```python
from build123d import *

# Parameters (mm, degrees)
GEARFACEPROFILE_R        = 15
GEARFACEEXTRUDE_DEPTH    = 12.21
CENTERSLOT_DEPTH         = 25.476194557
GEARCONNECTORS_OUTLINE_R = 3.5
GEARCONNECTORS_DEPTH     = 3.8
SETSCREWPROFILE_R        = 2.52
SETSCREWHOLE_DEPTH       = 25.476194557


# Read off the part's stored shape, not the designer's step: GearConnectors
with BuildPart() as part:
    # GearFaceProfile → GearFaceExtrude (new body)
    with BuildSketch(Plane.XY):
        Circle(GEARFACEPROFILE_R)
    extrude(amount=GEARFACEEXTRUDE_DEPTH)

    # Sketch1 → CenterSlot (cut, through all)
    with BuildSketch(Plane.XY.offset(12.21)):
        with BuildLine():
            Line((-1.335, 6.504411964), (-1.335, 4.704411964))
            Line((-1.335, 4.704411964), (1.335, 4.704411964))
            Line((1.335, 4.704411964), (1.335, 6.504411964))
            ThreePointArc((1.335, 6.504411964), (0, -6.64), (-1.335, 6.504411964))
        make_face()
    extrude(amount=-CENTERSLOT_DEPTH, mode=Mode.SUBTRACT)

    # GearConnectors outline → GearConnectors (add)
    with BuildSketch(Plane(origin=(0, 0, 0), x_dir=(-1, 0, 0), z_dir=(0, 0, -1))):
        with BuildLine():
            ThreePointArc((5.310262334, -3.986315836), (11.691342952, -6.749999998), (6.107381948, -2.605664164))
            ThreePointArc((6.107381948, -2.605664164), (5.750408681, -3.32), (5.310262334, -3.986315836))
        make_face()
        with BuildLine():
            ThreePointArc((-6.107381948, -2.605664164), (-11.691342952, -6.749999998), (-5.310262334, -3.986315836))
            ThreePointArc((-5.310262334, -3.986315836), (-5.750408681, -3.32), (-6.107381948, -2.605664164))
        make_face()
        with Locations((0, 10)):
            Circle(GEARCONNECTORS_OUTLINE_R)
    extrude(amount=GEARCONNECTORS_DEPTH)

    # SetScrewProfile → SetScrewHole (cut, through all)
    with BuildSketch(Plane(origin=(0, 0, 0), x_dir=(0, 0, -1), z_dir=(1, 0, 0))):
        with Locations((-6.105, 0)):
            Circle(SETSCREWPROFILE_R)
    extrude(amount=-SETSCREWHOLE_DEPTH, mode=Mode.SUBTRACT)


solid = part.part
```
Here's how the part is built. I have some questions about the finished solid (model axes, mm). A direction names the side the tool comes from. Round coordinates to 2 decimals unless told otherwise and drop trailing zeros. Loops run counter-clockwise (first coordinate to the right, second up) from the corner with the lowest first, then second, coordinate; pieces in that order, holes last. Notation, with made-up numbers: (16.25, 73.25) -> (53.25, 73.25) arc R18 cw to (53.25, 94.25) -> close; hole circle Ø7 at (-37, 63.5). An arc over 180 degrees is marked (long way). Answer as CSV lines item,"result".
1. If we section it at A-A on y = 0: Please give me the cut outline in (x, z) (3 decimals).
Final values:
outline,"(-15, 0) -> (-6.64, 0) -> (-6.64, 3.585) -> (-15, 3.585) -> close; (-15, 8.625) -> (-6.64, 8.625) -> (-6.64, 12.21) -> (-15, 12.21) -> close; (6.64, 0) -> (15, 0) -> (15, 12.21) -> (6.64, 12.21) -> close"
2. If we section it at D-D on y = -5: Please give me the cut outline in (x, z), plus the area to 3 significant figures.
Final values:
outline,"(-14.14, 0) -> (-12.16, 0) -> (-12.16, -3.8) -> (-5.16, -3.8) -> (-5.16, 0) -> (-4.37, 0) -> (-4.37, 12.21) -> (-14.14, 12.21) -> close; (4.37, 0) -> (5.16, 0) -> (5.16, -3.8) -> (12.16, -3.8) -> (12.16, 0) -> (14.14, 0) -> (14.14, 12.21) -> (4.37, 12.21) -> close"
area,"292 mm^2"
3. If I drill on L1, parallel to Z at x = -11, y = 0 (3 decimals); L2, parallel to X at y = 3, z = 3.75; L3, parallel to Z at x = -4, y = 13, over which ranges is the centre line in solid material (lowest first)?
Final values:
L1,"z = 0 to 3.585, 8.625 to 12.21"
L2,"x = -14.7 to -5.92, 5.92 to 14.7"
L3,"z = 0 to 12.21"
4. Which directions (+Z, -Z, +X, -X, +Y, -Y) give clear straight access to the entire face, cutting with the end or side of a thin tool? Please do faces 4 (the face through (3.1, -6.5, 12.21)), 5 (the face through (0, 4.704, 6)), 6 (the face through (0.759, 6.583, -1.873)).
Final values:
face 4,"+Z, +X, -X, +Y, -Y"
face 5,"+Z, -Z"
face 6,"-Z"
5. For pin 1 (2 mm diameter, centred on y = 5.5, z = 7.5, fed in from -X); pin 2 (0.5 mm diameter, centred on y = 6, z = 8.5, fed in from +X); pin 3 (5 mm diameter, centred on x = 11, z = 2, fed in from -Y), each with a flat end and sliding along its axis, tell me the tip position at first contact or that it passes through.
Final values:
pin 1,"stops at x = -14.31"
pin 2,"stops at x = 13.85"
pin 3,"stops at y = -12.36"
6. If we section it at B-B on x = 0: Please give me the cut outline in (y, z).
Final values:
outline,"(-15, 0) -> (-6.64, 0) -> (-6.64, 12.21) -> (-15, 12.21) -> close; (4.7, 0) -> (6.5, 0) -> (6.5, -3.8) -> (13.5, -3.8) -> (13.5, 0) -> (15, 0) -> (15, 12.21) -> (4.7, 12.21) -> close"
7. If we section it at C-C on z = -0.5: Please give me the cut outline in (x, y).
Final values:
outline,"(-6.11, -2.61) arc R3.5 ccw (long way) to (-5.31, -3.99) arc R6.64 cw to start; circle Ø7 at (0, 10); (5.31, -3.99) arc R3.5 ccw (long way) to (6.11, -2.61) arc R6.64 cw to start"
8. Thinking about a two-plate mould opening in Y: for faces 1 (the face through (-10.51, -2.46, 6.65)), 2 (the face through (-7, 0, 0)), 3 (the face through (13.856, -5.745, 6.02)), which applies, released by +Y, released by -Y, zero draft, split by the parting line, or undercut?
Final values:
face 1,"undercut"
face 2,"zero draft"
face 3,"split by the parting line"
